Could you check a few things on this model? Use its own coordinates, in mm. A direction names the side the tool comes from. Give positions to 0.01 mm unless a question says otherwise; leave off trailing zeros. Loops run counter-clockwise (first coordinate to the right, second up) from the corner with the lowest first, then second, coordinate; pieces in that order, holes last. Notation, with made-up numbers: (74, 87.25) - (100, 87.25) arc R12 cw to (100, 106.25) - close; hole circle Ø4 at (40.25, -36). An arc over 180 degrees is marked (long way). Write each question's results on one line, items separated by ' | '. Start each with the question number.
Autodesk Inventor part; units mm, degrees
ref_plane "YZ Plane" through (0, 0, 0) normal (1, 0, 0) x (0, 1, 0)
ref_plane "XZ Plane" through (0, 0, 0) normal (0, 1, 0) x (-1, 0, 0)
ref_plane "XY Plane" through (0, 0, 0) normal (0, 0, 1) x (1, 0, 0)
sketch "Boceto1" plane through (0, 0, 0) normal (0, 0, 1) x (1, 0, 0)
  circle A0 centre (0, 0) radius 4.5
  circle A1 centre (0, 0) radius 45
  dimension "d0" = 9
  dimension "d1" = 90
extrude "Extrusión1" add sketch "Boceto1" along normal blind 15
sketch "Boceto2" plane through (0, 0, 0) normal (0, 0, -1) x (-1, 0, 0)
  arc A0 (-6.9941, 2.7079) -> (-6.9941, -2.7079) centre (0, 0) ccw
  arc A1 (-33.0366, 17.7436) -> (-33.0366, -17.7436) centre (0, 0) ccw
  line L0 (-6.9941, 2.7079) -> (-33.0366, 17.7436)
  line L1 (-6.9941, -2.7079) -> (-33.0366, -17.7436)
  line L2 (-2.7079, -6.9941) -> (-17.7436, -33.0366)
  arc A2 (-17.7436, -33.0366) -> (17.7436, -33.0366) centre (0, 0) ccw
  line L3 (2.7079, -6.9941) -> (17.7436, -33.0366)
  arc A3 (-2.7079, -6.9941) -> (2.7079, -6.9941) centre (0, 0) ccw
  line L4 (6.9941, -2.7079) -> (33.0366, -17.7436)
  arc A4 (33.0366, -17.7436) -> (33.0366, 17.7436) centre (0, 0) ccw
  line L5 (6.9941, 2.7079) -> (33.0366, 17.7436)
  arc A5 (6.9941, -2.7079) -> (6.9941, 2.7079) centre (0, 0) ccw
  line L6 (2.7079, 6.9941) -> (17.7436, 33.0366)
  arc A6 (17.7436, 33.0366) -> (-17.7436, 33.0366) centre (0, 0) ccw
  line L7 (-2.7079, 6.9941) -> (-17.7436, 33.0366)
  arc A7 (2.7079, 6.9941) -> (-2.7079, 6.9941) centre (0, 0) ccw
  dimension "d4" = 15
  dimension "d5" = 75
  dimension "d13" = 360
extrude "Extrusión2" cut sketch "Boceto2" against normal through all
Q1. Which directions (+Z, -Z, +X, -X, +Y, -Y) give clear straight access to the entire face, cutting with the end or side of a thin tool? Please do faces 1 (the face through (0, 7.5, 7.4)), 2 (the face through (9, -9, 15)).
Q2. I want a section at C-C, the plane z = 12.75. List the corners of the cut face in (x, y) for me.
Q3. I need wall thicknesses on L1, parallel to Y at x = 0, z = 7.5; L2, parallel to X at y = -6, z = 7; L3, parallel to X at y = 5.5, z = 7. Which ranges of each line are inside material? Lowest first, please. Write a range as from..to.
Q4. I want a section at D-D, the plane y = 28.5. List the corners of the cut face in (x, z) for me.
Q5. I want a section at A-A, the plane y = 0. List the corners of the cut face in (x, z) for me.
Q6. I'm going to push flat-ended pins straight in: pin 1 Ø2 at (x, y) = (14.5, -34) entering from +Z; pin 2 Ø4 at (y, z) = (-14, 8.5) entering from +X; pin 3 Ø1.5 at (x, z) = (-21, 11.5) entering from -Y; pin 4 Ø2 at (y, z) = (20, 8) entering from -X. Where does each tip first touch, or does it pass through?
Q7. If we mould it in two halves opening along X, with no side actions, what happens to faces 3 (the face through (0.3, -37.5, 7.4)), 4 (the face through (9, -9, 0)), 5 (the face through (20.765, 39.923, 7.395))? For each: +X half, -X half, draft (parallel to the pull), parting line (faces both ways), or undercut.
Conclusion:
1) face 1: +Z, -Z | face 2: +Z, +X, -X, +Y, -Y
2) outline: circle Ø90 at (0, 0); hole (-33.04, -17.74) - (-6.99, -2.71) arc R7.5 cw to (-6.99, 2.71) - (-33.04, 17.74) arc R37.5 ccw to start; hole (-17.74, -33.04) arc R37.5 ccw to (17.74, -33.04) - (2.71, -6.99) arc R7.5 cw to (-2.71, -6.99) - close; hole (-17.74, 33.04) - (-2.71, 6.99) arc R7.5 cw to (2.71, 6.99) - (17.74, 33.04) arc R37.5 ccw to start; hole circle Ø9 at (0, 0); hole (6.99, -2.71) - (33.04, -17.74) arc R37.5 ccw to (33.04, 17.74) - (6.99, 2.71) arc R7.5 cw to start
3) L1: -45..-37.5, -7.5..-4.5, 4.5..7.5, 37.5..45 | L2: -44.6..-37.02, -12.7..12.7, 37.02..44.6 | L3: -44.66..-37.09, -11.83..11.83, 37.09..44.66
4) outline: (-34.82, 0) - (-15.12, 0) - (-15.12, 15) - (-34.82, 15) - close; (15.12, 0) - (34.82, 0) - (34.82, 15) - (15.12, 15) - close
5) outline: (-45, 0) - (-37.5, 0) - (-37.5, 15) - (-45, 15) - close; (-7.5, 0) - (-4.5, 0) - (-4.5, 15) - (-7.5, 15) - close; (4.5, 0) - (7.5, 0) - (7.5, 15) - (4.5, 15) - close; (37.5, 0) - (45, 0) - (45, 15) - (37.5, 15) - close
6) pin 1: z = 15 | pin 2: x = 43.37 | pin 3: y = -40.19 | pin 4: x = -40.79
7) face 3: undercut | face 4: draft | face 5: parting line
